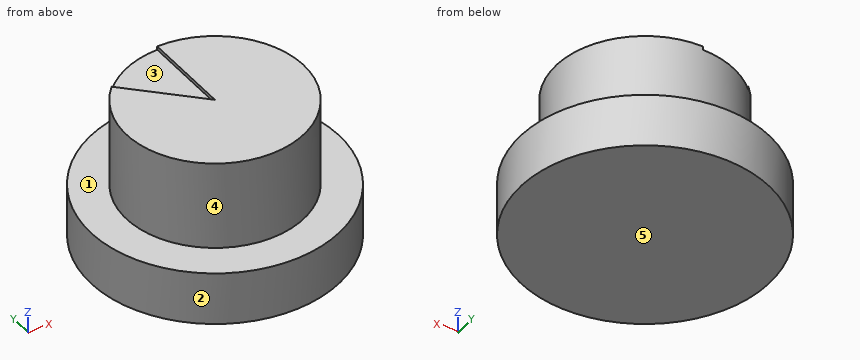
Autodesk Inventor part; units mm, degrees
ref_plane "YZ Plane" through (0, 0, 0) normal (1, 0, 0) x (0, 1, 0)
ref_plane "XZ Plane" through (0, 0, 0) normal (0, 1, 0) x (-1, 0, 0)
ref_plane "XY Plane" through (0, 0, 0) normal (0, 0, 1) x (1, 0, 0)
sketch "Sketch1" plane through (0, 0, 0) normal (0, 0, 1) x (1, 0, 0)
  circle A0 centre (0, 0) radius 7
  dimension "d0" = 14
extrude "Extrusion1" add sketch "Sketch1" along normal blind 3
sketch "Sketch2" plane through (0, 0, 3) normal (0, 0, 1) x (1, 0, 0)
  circle A0 centre (0, 0) radius 5
  dimension "d3" = 10
extrude "Extrusion2" add sketch "Sketch2" along normal blind 5
sketch "Sketch3" plane through (0, 0, 8) normal (0, 0, 1) x (1, 0, 0)
  circle A0 centre (0, 0) radius 5
  arc A1 (0.0676, 4.9995) -> (-3.4874, 3.583) centre (0, 0) ccw
  line L0 (0, 0) -> (0.0676, 4.9995)
  line L1 (0, 0) -> (-3.4874, 3.583)
  dimension "d6" = 45
extrude "Extrusion3" cut sketch "Sketch3" against normal blind 0.2 contours L0 L1 A0 picked at (-0.9199, 3.1872)
properties part number "potentiometer knob"
Could you check a few things on this model? Use its own coordinates, in mm. Face numbers are marked on the shaded views. A direction names the side the tool comes from. Coordinates: 2 decimals unless noted, no trailing zeros. Write each loop counter-clockwise with the first axis right and the second up, starting at its lowest first coordinate (ties: lowest second). Pieces come first, ordered by that corner, then holes. Notation, with made-up numbers: (22, 8) -> (50, 8) arc R13 cw to (50, 23) -> close; hole circle Ø10 at (32.25, 52). An arc over 180 degrees is marked (long way). Return JSON: item names as keys, results as strings.
(1) Imagine slicing it at C-C, the plane z = 2.25. Please give me the cut outline in (x, y).
Numbers:
{"outline": "circle Ø14 at (0, 0)"}
(2) I need wall thicknesses on L1, parallel to Z at x = -2, y = 6; L2, parallel to X at y = -4.5, z = 1; L3, parallel to Y at x = 0, z = 3.5. Which ranges of each line are inside material? Lowest first, please.
Numbers:
{"L1": "z = 0 to 3", "L2": "x = -5.36 to 5.36", "L3": "y = -5 to 5"}
(3) I'm going to push flat-ended pins straight in: pin 1 (3 mm diameter, centred on y = -1, z = 7, fed in from +X); pin 2 (4 mm diameter, centred on y = 4, z = 7, fed in from -X). Where does each tip first touch, or does it pass through?
Numbers:
{"pin 1": "stops at x = 5", "pin 2": "stops at x = -4.58"}
(4) Imagine slicing it at A-A, the plane y = 4.5. Please give me the cut outline in (x, z), then the cut area to 3 significant figures.
Numbers:
{"outline": "(-5.36, 0) -> (5.36, 0) -> (5.36, 3) -> (2.18, 3) -> (2.18, 8) -> (0.06, 8) -> (0.06, 7.8) -> (-2.18, 7.8) -> (-2.18, 3) -> (-5.36, 3) -> close", "area": "53.5 mm2"}
(5) We'd pull the mould along X, two halves only. Please class the marked faces 3, 4 and 5: +X half, -X half, draft (parallel to the pull), parting line (faces both ways), or undercut.
Numbers:
{"face 3": "undercut", "face 4": "parting line", "face 5": "draft"}
(6) Imagine slicing it at D-D, the plane x = 1.5. Please give me the cut outline in (y, z), then the cut area to 3 significant figures.
Numbers:
{"outline": "(-6.84, 0) -> (6.84, 0) -> (6.84, 3) -> (4.77, 3) -> (4.77, 8) -> (-4.77, 8) -> (-4.77, 3) -> (-6.84, 3) -> close", "area": "88.7 mm2"}
(7) Which directions (+Z, -Z, +X, -X, +Y, -Y) give clear straight access to the entire face, cutting with the end or side of a thin tool? Please do the marked faces 1 and 2.
Numbers:
{"face 1": "+Z", "face 2": "+Z, -Z"}
(8) Imagine slicing it at B-B, the plane x = -3. Please give me the cut outline in (y, z), then the cut area to 3 significant figures.
Numbers:
{"outline": "(-6.32, 0) -> (6.32, 0) -> (6.32, 3) -> (4, 3) -> (4, 7.8) -> (3.08, 7.8) -> (3.08, 8) -> (-4, 8) -> (-4, 3) -> (-6.32, 3) -> close", "area": "77.8 mm2"}
